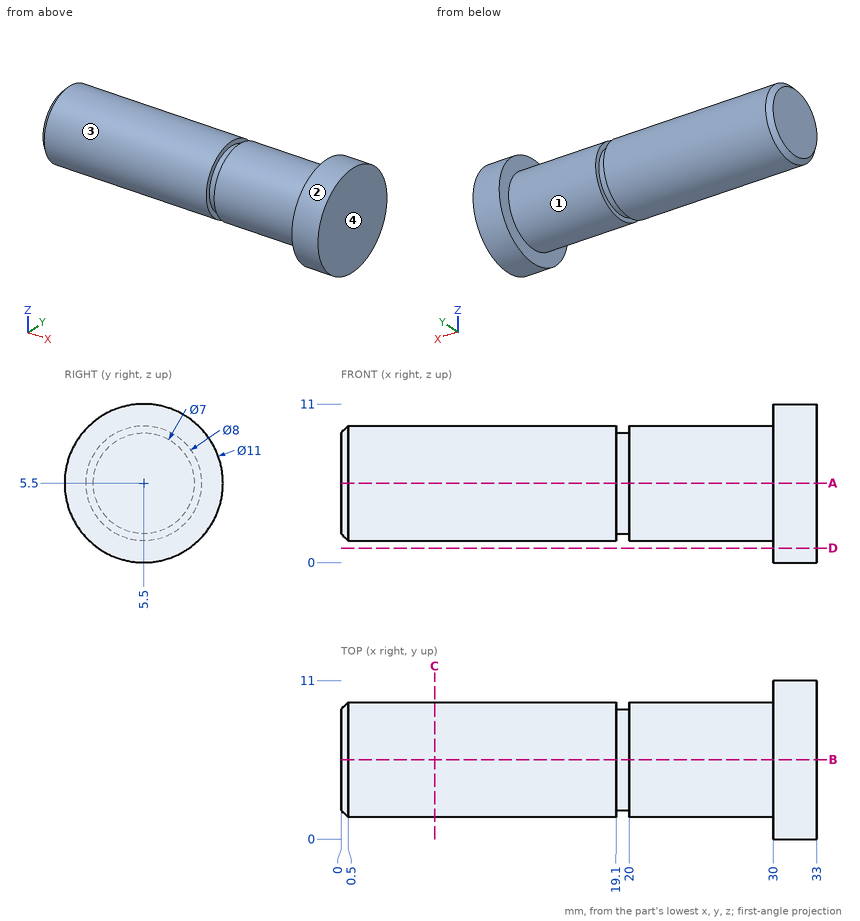
Study the drawing (mm; zero at the part's minimum x, y, z) and answer. A direction names the side the tool comes from. Round coordinates to 2 decimals unless told otherwise and drop trailing zeros. Write each loop counter-clockwise with the first axis right and the second up, starting at its lowest first coordinate (ties: lowest second). Pieces come first, ordered by that corner, then holes. Notation, with made-up numbers: (63, 31) - (85, 31) arc R33 cw to (85, 64) - close; hole circle Ø10 at (14.25, 13.5). An arc over 180 degrees is marked (long way). Return JSON: item names as keys, results as strings. Group by question number.
Q1. The part is cut by section D-D on z = 1. Write down the section's boundary in (x, y), then the cut area to 3 significant figures.
Q2. The mould has two halves that part along Y. Classify the marked faces 3 and 4: released by +Y, released by -Y, zero draft, split by the parting line, or undercut.
Q3. The part is cut by section C-C on x = 6.5. Write down the section's boundary in (y, z).
Q4. The part is cut by section A-A on z = 5.5. Write down the section's boundary in (x, y).
Q5. Each of these flat-tipped pins is pushed along its axis until it touches: pin 1 Ø5.5 at (y, z) = (6.5, 7.5) entering from -X; pin 2 Ø3 at (x, z) = (9.5, 7) entering from +Y; pin 3 Ø5 at (x, z) = (15, 8.5) entering from -Y; pin 4 Ø6 at (x, y) = (18, 1.5) entering from +Z. Where does it stop, or does it pass through?
Q6. For the marked faces 1 and 2, determine the directions among +Z, -Z, +X, -X, +Y, -Y from which every point of the face is accessible in a straight line to the end or side of a thin tool.
Q7. Find the intervals of material crossed by L1, parallel to Y at x = 22, z = 5.25; L2, parallel to X at y = 3, z = 1; L3, parallel to Y at x = 19.5, z = 5.5, in increasing order.
Solved:
{
 "1": {"outline": "(30, 2.34) - (33, 2.34) - (33, 8.66) - (30, 8.66) - close", "area": "19.0 mm²"},
 "2": {"face 3": "split by the parting line", "face 4": "zero draft"},
 "3": {"outline": "circle Ø8 at (5.5, 5.5)"},
 "4": {"outline": "(0, 2) - (0.5, 1.5) - (19.1, 1.5) - (19.1, 2) - (20, 2) - (20, 1.5) - (30, 1.5) - (30, 0) - (33, 0) - (33, 11) - (30, 11) - (30, 9.5) - (20, 9.5) - (20, 9) - (19.1, 9) - (19.1, 9.5) - (0.5, 9.5) - (0, 9) - close"},
 "5": {"pin 1": "x = 0", "pin 2": "y = 9.5", "pin 3": "y = 1.53", "pin 4": "z = 9.37"},
 "6": {"face 1": "-X", "face 2": "+X, -X"},
 "7": {"L1": "1.51 to 9.49", "L2": "30 to 33", "L3": "2 to 9"}
}
